Build history of the part. All positions in model axes, mm. Face numbers are marked on the shaded views. A direction names the side the tool comes from. Round coordinates to 2 decimals unless told otherwise and drop trailing zeros. Write each loop counter-clockwise with the first axis right and the second up, starting at its lowest first coordinate (ties: lowest second). Pieces come first, ordered by that corner, then holes. Notation, with made-up numbers: (72, 69.5) -> (116, 69.5) arc R14 cw to (116, 91.5) -> close; hole circle Ø2 at (-34, -2.5). An arc over 180 degrees is marked (long way). Return JSON: item names as keys, results as strings.
from build123d import *

# Parameters (mm, degrees)
SKETCH_W     = 52
SKETCH_H     = 18
PAD_DEPTH    = 7
SKETCH001_W  = 52
SKETCH001_H  = 5
PAD001_DEPTH = 25
SKETCH002_R  = 1.8
SKETCH002_W  = 12
SKETCH002_H  = 18
POCKET_DEPTH = 5


with BuildPart() as part:
    # Sketch → Pad (new body)
    with BuildSketch(Plane.XY):
        with Locations((0, -7)):
            Rectangle(SKETCH_W, SKETCH_H)
    extrude(amount=PAD_DEPTH)

    # Sketch001 → Pad001 (new body)
    with BuildSketch(Plane.XY.offset(7)):
        with Locations((0, -2.5)):
            Rectangle(SKETCH001_W, SKETCH001_H)
    extrude(amount=PAD001_DEPTH)

    # Sketch002 → Pocket (cut)
    with BuildSketch(Plane.XZ.offset(5)):
        with Locations((-18.5, 14.5)):
            Circle(SKETCH002_R)
        with Locations((18.5, 14.5)):
            Circle(SKETCH002_R)
        with Locations((0, 16)):
            Rectangle(SKETCH002_W, SKETCH002_H)
        Polygon((-26, 14), (-6, 32), (-26, 32), align=None)
        Polygon((6, 32), (26, 14), (26, 32), align=None)
    extrude(amount=-POCKET_DEPTH, mode=Mode.SUBTRACT)


solid = part.part
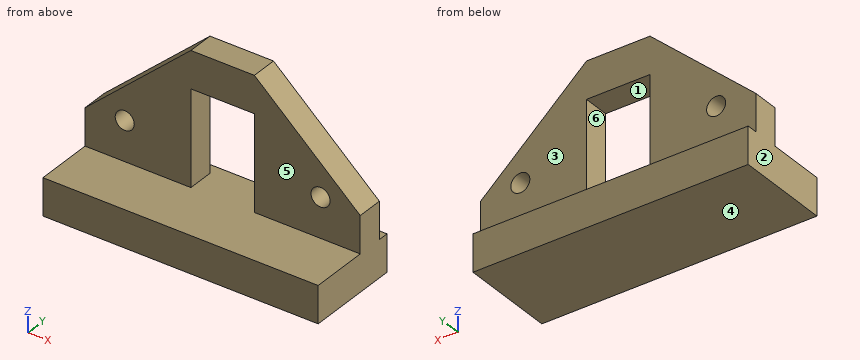
Q1. Two-plate mould, pull along Z, no slides. Class the marked faces 4, 5 and 6: +Z half, -Z half, draft (parallel to the pull), parting line (faces both ways), or undercut.
Verdict:
{"face 4": "-Z half", "face 5": "draft", "face 6": "undercut"}
Q2. 3-axis set-ups, long thin cutter, end or side, ignore diameter. For the marked faces 1, 2 and 3: which of +Z, -Z, +X, -X, +Y, -Y reach the whole face in a straight line?
Verdict:
{"face 1": "+Y, -Y", "face 2": "+Z, -Z, -X, +Y, -Y", "face 3": "+Z, +X, -X, +Y"}
Q3. Saw through at C-C on y = -1. List the corners of the cut face in (x, z).
Verdict:
{"outline": "(-26, 0) -> (26, 0) -> (26, 14) -> (6, 32) -> (-6, 32) -> (-26, 14) -> close; hole circle Ø3.6 at (-18.5, 14.5); hole (-6, 7) -> (6, 7) -> (6, 25) -> (-6, 25) -> close; hole circle Ø3.6 at (18.5, 14.5)"}
Q4. Saw through at B-B on z = 12. List the corners of the cut face in (x, y).
Verdict:
{"outline": "(-26, -5) -> (-6, -5) -> (-6, 0) -> (-26, 0) -> close; (6, -5) -> (26, -5) -> (26, 0) -> (6, 0) -> close"}
Q5. Wall check: L1, parallel to Z at x = 2.5, y = -8.25; L2, parallel to Y at x = -4, z = 29.5; L3, parallel to Z at x = -18.5, y = -3.1. Give the ranges that are in metal, low to high.
Verdict:
{"L1": "z = 0 to 7", "L2": "y = -5 to 0", "L3": "z = 0 to 12.7, 16.3 to 20.75"}
Q6. Saw through at D-D on x = 11.5. List the corners of the cut face in (y, z).
Verdict:
{"outline": "(-16, 0) -> (2, 0) -> (2, 7) -> (0, 7) -> (0, 27.05) -> (-5, 27.05) -> (-5, 7) -> (-16, 7) -> close"}
Q7. Pin check, flat tips, straight feed: pin 1 Ø4 at (x, z) = (-9, 20.5) entering from -Y; pin 2 Ø8 at (x, z) = (-2.5, 23.5) entering from +Y; pin 3 Ø8 at (x, y) = (-16, -9.5) entering from +Z; pin 4 Ø8 at (x, z) = (19.5, 28) entering from -Y. Stop position of each tip, or through.
Verdict:
{"pin 1": "stops at y = -5", "pin 2": "stops at y = 0", "pin 3": "stops at z = 7", "pin 4": "passes through"}
Q8. Saw through at A-A on x = 18.5. List the corners of the cut face in (y, z).
Verdict:
{"outline": "(-16, 0) -> (2, 0) -> (2, 7) -> (0, 7) -> (0, 12.7) -> (-5, 12.7) -> (-5, 7) -> (-16, 7) -> close; (-5, 16.3) -> (0, 16.3) -> (0, 20.75) -> (-5, 20.75) -> close"}
